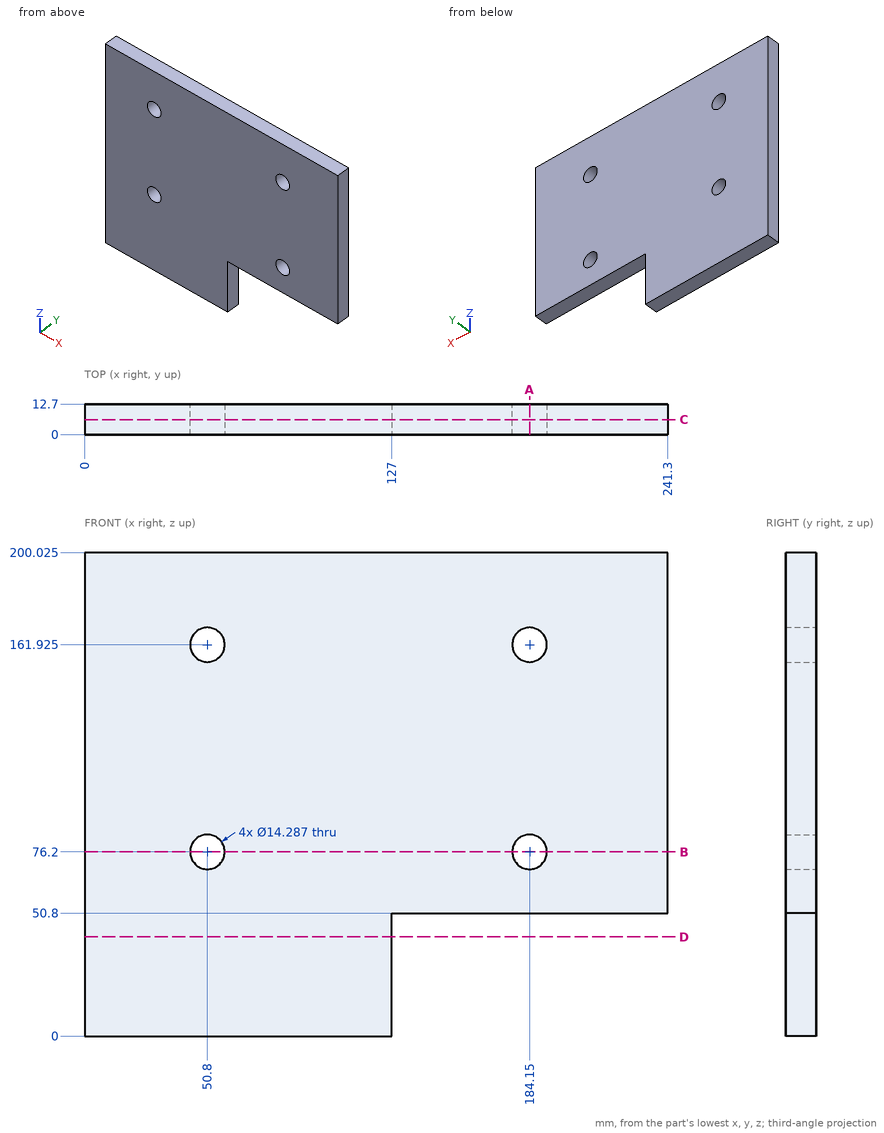
Job drawing, mm, ordinate dimensions from the low corner. One solid piece. Coordinates: 2 decimals unless noted, no trailing zeros. Loops run counter-clockwise (first coordinate to the right, second up) from the corner with the lowest first, then second, coordinate; pieces in that order, holes last. Notation, with made-up numbers: (24, -12.5) - (83, -12.5) arc R28 cw to (83, 5.5) - close; hole circle Ø9 at (-37, 27). An arc over 180 degrees is marked (long way). Write item = value, one per line. Start each with the question number.
Q1. Drill centre lines: L1, parallel to Z at x = 50.8, y = 8.5 (1 decimal); L2, parallel to Z at x = 184.15, y = 2.5 (1 decimal); L3, parallel to Z at x = 138, y = 11.5 (1 decimal). Where is each one in solid material? Low to high.
Q2. Cut at B-B, the plane z = 76.2. List the corners of the cut face in (x, y), then the cut area to 3 significant figures.
Q3. Cut at A-A, the plane x = 184.15. List the corners of the cut face in (y, z) (1 decimal).
Q4. Cut at C-C, the plane y = 6.25. Give the number of separate pieces and of enclosed holes in the cut face, then the cut area to 3 significant figures.
Q5. Flat gauge pins, fed straight in: pin 1 Ø16.5 at (x, z) = (50.8, 161.925) entering from -Y; pin 2 Ø4 at (x, y) = (193, 5.5) entering from -Z; pin 3 Ø13 at (x, z) = (50.8, 76.2) entering from -Y. Where does each tip first touch, or does it go through?
Q6. Cut at D-D, the plane z = 41. List the corners of the cut face in (x, y).
Computed:
q1.L1 = 0 to 69.1, 83.3 to 154.8, 169.1 to 200
q1.L2 = 50.8 to 69.1, 83.3 to 154.8, 169.1 to 200
q1.L3 = 50.8 to 200
q2.outline = (0, 0) - (43.66, 0) - (43.66, 12.7) - (0, 12.7) - close; (57.94, 0) - (177.01, 0) - (177.01, 12.7) - (57.94, 12.7) - close; (191.29, 0) - (241.3, 0) - (241.3, 12.7) - (191.29, 12.7) - close
q2.area = 2,700 mm²
q3.outline = (0, 50.8) - (12.7, 50.8) - (12.7, 69.1) - (0, 69.1) - close; (0, 83.3) - (12.7, 83.3) - (12.7, 154.8) - (0, 154.8) - close; (0, 169.1) - (12.7, 169.1) - (12.7, 200) - (0, 200) - close
q4.separate_pieces = 1
q4.enclosed_holes = 4
q4.area = 41,800 mm²
q5.pin_1 = 0
q5.pin_2 = 50.8
q5.pin_3 = through
q6.outline = (0, 0) - (127, 0) - (127, 12.7) - (0, 12.7) - close
